Work out the finished part from the listing and answer in its coordinate system (mm). A direction names the side the tool comes from. Give positions to 0.01 mm unless a question says otherwise; leave off trailing zeros. Loops run counter-clockwise (first coordinate to the right, second up) from the corner with the lowest first, then second, coordinate; pieces in that order, holes last.
from build123d import *

# Parameters (mm, degrees)
SKETCH1_W           = 120
SKETCH1_H           = 48
BOSS_EXTRUDE1_DEPTH = 40
SKETCH3_W           = 104
SKETCH3_H           = 42
CUT_EXTRUDE1_DEPTH  = 37
CUT_EXTRUDE2_DEPTH  = 37
CUT_EXTRUDE4_DEPTH  = 110
SKETCH10_W          = 48
SKETCH10_H          = 5
BOSS_EXTRUDE3_DEPTH = 2
SKETCH11_W          = 30
SKETCH11_H          = 10
BOSS_EXTRUDE4_DEPTH = 10
CUT_EXTRUDE6_DEPTH  = 8
FILLET1_R           = 2
CUT_EXTRUDE5_DEPTH  = 110


with BuildPart() as part:
    # Sketch1 → Boss-Extrude1 (new body)
    with BuildSketch(Plane(origin=(0, 0, 0), x_dir=(1, 0, 0), z_dir=(0, 1, 0))):
        with Locations((60, 24)):
            Rectangle(SKETCH1_W, SKETCH1_H)
    extrude(amount=BOSS_EXTRUDE1_DEPTH)

    # Sketch3 → Cut-Extrude1 (cut)
    with BuildSketch(Plane(origin=(0, 40, 0), x_dir=(1, 0, 0), z_dir=(0, 1, 0))):
        with Locations((58, 24)):
            Rectangle(SKETCH3_W, SKETCH3_H)
    extrude(amount=-CUT_EXTRUDE1_DEPTH, mode=Mode.SUBTRACT)

    # Sketch5 → Cut-Extrude2 (cut)
    with BuildSketch(Plane(origin=(0, 3, 0), x_dir=(1, 0, 0), z_dir=(0, 1, 0))):
        with BuildLine():
            Line((11, 42), (105, 42))
            ThreePointArc((105, 42), (106, 41), (105, 40))
            Line((105, 40), (11, 40))
            ThreePointArc((11, 40), (10, 41), (11, 42))
        make_face()
        with BuildLine():
            Line((11, 35.1), (105, 35.1))
            ThreePointArc((105, 35.1), (106, 36.1), (105, 37.1))
            Line((105, 37.1), (11, 37.1))
            ThreePointArc((11, 37.1), (10, 36.1), (11, 35.1))
        make_face()
        with BuildLine():
            Line((11, 30.2), (105, 30.2))
            ThreePointArc((105, 30.2), (106, 31.2), (105, 32.2))
            Line((105, 32.2), (11, 32.2))
            ThreePointArc((11, 32.2), (10, 31.2), (11, 30.2))
        make_face()
        with BuildLine():
            Line((11, 25.3), (105, 25.3))
            ThreePointArc((105, 25.3), (106, 26.3), (105, 27.3))
            Line((105, 27.3), (11, 27.3))
            ThreePointArc((11, 27.3), (10, 26.3), (11, 25.3))
        make_face()
        with BuildLine():
            Line((11, 20.4), (105, 20.4))
            ThreePointArc((105, 20.4), (106, 21.4), (105, 22.4))
            Line((105, 22.4), (11, 22.4))
            ThreePointArc((11, 22.4), (10, 21.4), (11, 20.4))
        make_face()
        with BuildLine():
            Line((11, 15.5), (105, 15.5))
            ThreePointArc((105, 15.5), (106, 16.5), (105, 17.5))
            Line((105, 17.5), (11, 17.5))
            ThreePointArc((11, 17.5), (10, 16.5), (11, 15.5))
        make_face()
        with BuildLine():
            Line((11, 10.6), (105, 10.6))
            ThreePointArc((105, 10.6), (106, 11.6), (105, 12.6))
            Line((105, 12.6), (11, 12.6))
            ThreePointArc((11, 12.6), (10, 11.6), (11, 10.6))
        make_face()
        with BuildLine():
            Line((11, 5.7), (105, 5.7))
            ThreePointArc((105, 5.7), (106, 6.7), (105, 7.7))
            Line((105, 7.7), (11, 7.7))
            ThreePointArc((11, 7.7), (10, 6.7), (11, 5.7))
        make_face()
    extrude(amount=-CUT_EXTRUDE2_DEPTH, mode=Mode.SUBTRACT)

    # Sketch7 → Cut-Extrude4 (cut)
    with BuildSketch(Plane.ZY):
        with BuildLine():
            Line((-2, 39.5), (-2, 40.5))
            ThreePointArc((-2, 40.5), (-1.5, 41), (-1, 40.5))
            Line((-1, 40.5), (-1, 39.5))
            ThreePointArc((-1, 39.5), (-1.5, 39), (-2, 39.5))
        make_face()
    cut_extrude4 = extrude(amount=-CUT_EXTRUDE4_DEPTH, mode=Mode.SUBTRACT)

    # Mirror1: Cut-Extrude4 across plane
    add(cut_extrude4.mirror(Plane(origin=(0, 0, -24), x_dir=(1, 0, 0), z_dir=(0, 0, -1))), mode=Mode.SUBTRACT)

    # Sketch10 → Boss-Extrude3 (add)
    with BuildSketch(Plane.ZY):
        with Locations((-24, 2.5)):
            Rectangle(SKETCH10_W, SKETCH10_H)
    extrude(amount=BOSS_EXTRUDE3_DEPTH)

    # Sketch11 → Boss-Extrude4 (add)
    with BuildSketch(Plane(origin=(120, 0, 0), x_dir=(0, 0, -1), z_dir=(1, 0, 0))):
        with Locations((24, 15)):
            Rectangle(SKETCH11_W, SKETCH11_H)
    extrude(amount=BOSS_EXTRUDE4_DEPTH)

    # Sketch12 → Cut-Extrude6 (cut)
    with BuildSketch(Plane(origin=(0, 20, 0), x_dir=(1, 0, 0), z_dir=(0, 1, 0))):
        with BuildLine():
            Line((128, 34), (128, 14))
            ThreePointArc((128, 14), (125, 11), (122, 14))
            Line((122, 14), (122, 34))
            ThreePointArc((122, 34), (125, 37), (128, 34))
        make_face()
    extrude(amount=-CUT_EXTRUDE6_DEPTH, mode=Mode.SUBTRACT)

    # Fillet1
    fillet1_edges = [part.edges().sort_by_distance(p)[0] for p in [
        (120, 15, -9),
        (125, 20, -9),
        (120, 10, -24),
        (125, 10, -9),
        (120, 15, -39),
        (125, 10, -39),
        (120, 20, -24),
        (125, 20, -39),
        (130, 15, -9),
        (130, 10, -24),
        (130, 15, -39),
        (130, 20, -24),
        (125, 12, -37),
        (128, 12, -24),
        (125, 12, -11),
        (122, 12, -24),
    ]]
    fillet(fillet1_edges, radius=FILLET1_R - 0.0001)  # a hair under: the kernel refuses the full size

    # Sketch8 → Cut-Extrude5 (cut)
    with BuildSketch(Plane.ZY.offset(2)):
        with BuildLine():
            Line((-48.5, 2), (-47.5, 2))
            ThreePointArc((-47.5, 2), (-47, 1.5), (-47.5, 1))
            Line((-47.5, 1), (-48.5, 1))
            ThreePointArc((-48.5, 1), (-49, 1.5), (-48.5, 2))
        make_face()
    extrude(amount=-CUT_EXTRUDE5_DEPTH, mode=Mode.SUBTRACT)


solid = part.part
Item 1: Find section C-C, the plane x = 76. Give the number of separate pieces and of enclosed holes in the cut face, plus the area to 3 significant figures.
Item 2: Determine the mould class of faces 1 (the face through (60, 20, -48)), 2 (the face through (-2, 3, -24)), 3 (the face through (57, 2, -25.3)) for opening direction X: released by +X, released by -X, zero draft, split by the parting line, or undercut.
Item 3: Find section A-A, the plane y = 32. Write down the section's boundary in (x, z).
Item 4: For faces 4 (the face through (60, 20, 0)), 5 (the face through (59, 2, -37.1)), 6 (the face through (125, 10, -24)), 7 (the face through (6, 22, -24)), determine the directions among +Z, -Z, +X, -X, +Y, -Y from which every point of the face is accessible in a straight line to the end or side of a thin tool.
Item 5: Flat-ended cylindrical pins translate along their axes: pin 1 Ø2 at (y, z) = (31, -39.5) entering from -X; pin 2 Ø1 at (x, z) = (97, -27) entering from +Y; pin 3 Ø6.5 at (x, z) = (124, -25.5) entering from +Y. Find the tip coordinate at first contact, or state that the pin passes through.
Item 6: Consider line 1 (Z direction, x = 48, y = 14); line 2 (X direction, y = 6, z = -16.5); line 3 (X direction, y = 3.5, z = -34). Determine where each line is inside the solid, lowest interval first.
Ans:
1. separate pieces: 9
1. enclosed holes: 0
1. area: 315 mm2
2. face 1: zero draft
2. face 2: released by -X
2. face 3: undercut
3. outline: (0, -48) - (120, -48) - (120, 0) - (0, 0) - close; hole (6, -45) - (110, -45) - (110, -3) - (6, -3) - close
4. face 4: +Z, +X, -X, +Y, -Y
4. face 5: +Y, -Y
4. face 6: +Z, -Z, +X, -Y
4. face 7: +Y
5. pin 1: stops at x = 0
5. pin 2: stops at y = 3
5. pin 3: stops at y = 20.44
6. line 1: z = -48 to -45, -3 to 0
6. line 2: x = 0 to 6, 110 to 120
6. line 3: x = -2 to 6, 110 to 120
